Autodesk Inventor part; units mm, degrees
ref_plane "YZ Plane" through (0, 0, 0) normal (1, 0, 0) x (0, 1, 0)
ref_plane "XZ Plane" through (0, 0, 0) normal (0, 1, 0) x (-1, 0, 0)
ref_plane "XY Plane" through (0, 0, 0) normal (0, 0, 1) x (1, 0, 0)
sketch "Szkic1" plane through (0, 0, 0) normal (0, 0, 1) x (1, 0, 0)
  circle A0 centre (0, 0) radius 50
  circle A1 centre (0, 0) radius 46
  circle A2 centre (0, 0) radius 31.5
  circle A3 centre (-28.9914, 28.9914) radius 3.4
  circle A4 centre (-28.9914, -28.9914) radius 3.4
  circle A5 centre (28.9914, 28.9914) radius 3.4
  circle A6 centre (28.9914, -28.9914) radius 3.4
  dimension "d0" = 100
  dimension "d1" = 92
  dimension "d2" = 63
  dimension "d4" = 6.8
  dimension "d5" = 6.8
  dimension "d6" = 6.8
  dimension "d7" = 6.8
extrude "Wyciągnięcie proste1" add sketch "Szkic1" along normal blind 4 contours A1
extrude "Wyciągnięcie proste2" add sketch "Szkic1" along normal blind 700 contours A0
sketch "Szkic5" plane through (0, 0, 0) normal (0, 1, 0) x (-1, 0, 0)
  line L0 (50, 700) -> (-50, 700)
  arc A0 (70, 700) -> (-70, 700) centre (0, 700) ccw
  circle A1 centre (0, 700) radius 26
  circle A2 centre (0, 700) radius 31
  line L1 (0, 630) -> (70, 630)
  line L2 (70, 630) -> (70, 700)
  line L3 (0, 630) -> (-70, 630)
  line L4 (-70, 630) -> (-70, 700)
  line L5 (0, 637.5) -> (70, 637.5)
  line L6 (0, 637.5) -> (-70, 637.5)
  point P0 (0, 0)
  point P1 (26, 700)
  point P2 (-26, 700)
  dimension "d28" = 140
  dimension "d29" = 52
  dimension "d35" = 62
extrude "Wyciągnięcie proste7" add sketch "Szkic5" along normal mid plane 130 contours A2 L0 A1 | L0 A1 A2 | A1 L0 | L0 A1 | L2 L5 L6 L4 A0 | L2 L1 L3 L4 L6 L5
extrude "Wyciągnięcie proste8" cut sketch "Szkic5" along normal mid plane 130 contours A1 L0 | L0 A1
extrude "Wyciągnięcie proste9" add sketch "Szkic5" along normal mid plane 150 contours A2 L0 A1 | L0 A1 A2
extrude "Wyciągnięcie proste10" cut sketch "Szkic5" along normal mid plane 118 contours A2 L0 A1 | L0 A1 A2 | A1 L0 | L0 A1 | L2 L5 L6 L4 A0 | L2 L1 L3 L4 L6 L5
sketch "Szkic7" plane through (0, 65, 700) normal (0, 1, 0) x (1, 0, 0)
  circle A0 centre (-48, 0) radius 7.5
  circle A1 centre (-48, 0) radius 12.5
  circle A2 centre (-48, 0) radius 15
  line L0 (-70, 70) -> (-70, 0)
  line L1 (-70, 70) -> (-94, 70)
  line L2 (-100, 64) -> (-100, -24)
  arc A3 (-70, 0) -> (70, 0) centre (0, 0) ccw
  line L3 (-94, -30) -> (-63.2456, -30)
  arc A4 (-100, -24) -> (-94, -30) centre (-94, -24) ccw
  arc A5 (-94, 70) -> (-100, 64) centre (-94, 64) ccw
  arc A6 (-80, 55) -> (-90, 55) centre (-85, 55) ccw
  arc A7 (-90, -15) -> (-80, -15) centre (-85, -15) ccw
  arc A8 (-90, 30) -> (-80, 30) centre (-85, 30) ccw
  arc A9 (-80, 10) -> (-90, 10) centre (-85, 10) ccw
  line L4 (-80, 10) -> (-80, -15)
  line L5 (-90, -15) -> (-90, 10)
  line L6 (-80, 55) -> (-80, 30)
  line L7 (-90, 30) -> (-90, 55)
  point P0 (0, 700)
  point P1 (-100, 70)
  point P2 (-100, -30)
  dimension "d46" = 15
  dimension "d47" = 25
  dimension "d48" = 30
  dimension "d57" = 30
  dimension "d58" = 100
  dimension "d59" = 6
  dimension "d60" = 6
  dimension "d62" = 10
  dimension "d63" = 10
  dimension "d64" = 10
  dimension "d66" = 10
  dimension "d67" = 25
extrude "Wyciągnięcie proste13" add sketch "Szkic7" along normal blind 10 contours A2
extrude "Wyciągnięcie proste14" cut sketch "Szkic7" against normal blind 6 contours A0
extrude "Wyciągnięcie proste15" add sketch "Szkic5" along normal mid plane 130 contours L2 L1 L3 L4 L6 L5
fillet "Zaokrąglenie1" radius 6 4 edges at (0, 65, 630) (0, -65, 630) (0, 59, 637.5) (0, -59, 637.5)
fillet "Zaokrąglenie2" radius 6 1 edges at (-50, 0, 630)
extrude "Wyciągnięcie proste16" add sketch "Szkic7" against normal blind 6 contours L0 A3 L3 A4 L2 A5 L1
thread "Gwint1"
thread "Gwint2"
thread "Gwint3"
thread "Gwint4"
thread "Gwint5"
properties part number "czlon_1" material "CFRP — polimer wzmocniony włóknem szklanym"
Design review of the part built by this model. Coordinates are the model's own, in mm. A direction names the side the tool comes from. Give positions to 0.01 mm unless a question says otherwise; leave off trailing zeros. Write each loop counter-clockwise with the first axis right and the second up, starting at its lowest first coordinate (ties: lowest second). Pieces come first, ordered by that corner, then holes. Notation, with made-up numbers: M 80.25,39.5 L 85.25,39.5 A9 cw 85.25,49.5 Z; hole C 26,-8.5 d3. An arc over 180 degrees is marked long. Answer as a JSON object with one key per item and string values. Group by question number.
1) For line 1 along X through (y, z) = (60, 700); line 2 along Z through (x, y) = (-48, 70); line 3 along X through (y, z) = (0, 466), list the stretches that pass through material, from the lowest coordinate up.
2) We need section C-C (x = 6). Count the separate pieces of the cut face and the enclosed holes in it, and give its area (3 significant figures).
3) We need section A-A (y = 0). Give the boundary of the cut face in (x, z), and give its area (3 significant figures).
4) Mouldability with a two-part tool opening along Z and no side actions: class faces 1 (the face through (16, -75, 679)), 2 (the face through (-50.71, 69.93, 687.797)), 3 (the face through (1.539, -62.042, 769.983)) as released by +Z, released by -Z, zero draft, split by the parting line, or undercut.
5) Tool access review of faces 4 (the face through (-30, -65, 689)), 5 (the face through (-51.252, 69.93, 685.357)), 6 (the face through (17, -59, 722)), 7 (the face through (47.69, -15.02, 307.63)): name each direction out of +Z, -Z, +X, -X, +Y, -Y from which nothing blocks a thin tool from reaching the whole face with its end or side.
6) Clearance check with flat-ended pins moving along their axes: pin 1 Ø5 at (x, y) = (-28.5, 48.5) entering from -Z; pin 2 Ø1.8 at (x, y) = (-87.5, 63) entering from -Z; pin 3 Ø10 at (x, z) = (14, 515.5) entering from +Y. State where each tip first meets the part, or that it passes through.
7) We need section B-B (z = 256). Give the boundary of the cut face in (x, y).
Answer key:
{
 "1": {"line 1": "x = -100 to -90, -80 to -55.5, -40.5 to -26, 26 to 70", "line 2": "z = 685 to 687.5, 712.5 to 715", "line 3": "x = -50 to -46, 46 to 50"},
 "2": {"separate pieces": "3", "enclosed holes": "0", "area": "7,370 mm²"},
 "3": {"outline": "M -70,630 L -56,630 A6 cw -50,624 L -50,0 L -31.5,0 L -31.5,4 L -46,4 L -46,630 L 46,630 L 46,4 L 31.5,4 L 31.5,0 L 50,0 L 50,624 A6 cw 56,630 L 70,630 L 70,637.5 L -70,637.5 Z", "area": "6,220 mm²"},
 "4": {"face 1": "zero draft", "face 2": "undercut", "face 3": "released by +Z"},
 "5": {"face 4": "-Y", "face 5": "+Y", "face 6": "+Z, +X, -X", "face 7": "-Z"},
 "6": {"pin 1": "stops at z = 629.56", "pin 2": "stops at z = 630", "pin 3": "stops at y = 49.18"},
 "7": {"outline": "C 0,0 d100; hole C 0,0 d92"}
}
